Source: CAD feature listing. Evaluate the final solid. Frame: model axes, mm. A direction names the side the tool comes from. Round coordinates to 2 decimals unless told otherwise and drop trailing zeros. Write each loop counter-clockwise with the first axis right and the second up, starting at its lowest first coordinate (ties: lowest second). Pieces come first, ordered by that corner, then holes. Notation, with made-up numbers: M 46.25,65.5 L 97.25,65.5 A26 ccw 97.25,88.5 Z; hole C -32.5,70.5 d9. An arc over 180 degrees is marked long. Answer in a Markdown table with one row per item.
from build123d import *

# Parameters (mm, degrees)
SKETCH1_W               = 59.992800004
SKETCH1_H               = 59.7535
BOSS_EXTRUDE1_DEPTH     = 2.54
SKETCH2_R               = 2.286000002
BOSS_EXTRUDE2_DEPTH     = 4.7625
SKETCH3_R               = 1.270000002
CUT_EXTRUDE1_DEPTH      = 3.175
CUT_EXTRUDE2_REACH      = 44.962
SKETCH4_W               = 30.1625
SKETCH4_H               = 22.225
CUT_EXTRUDE3_REACH      = 44.962
SKETCH5_R               = 1.269999998
SKETCH6_W               = 38.1
SKETCH6_H               = 1.5875
BOSS_EXTRUDE3_DEPTH     = 3.175
CHAMFER1_SIZE           = 3.175
CUT_EXTRUDE4_DEPTH      = 43.603821541
CUT_EXTRUDE4_DEPTH_BACK = 43.603821541
CUT_EXTRUDE5_DEPTH      = 9.525
CUT_EXTRUDE5_DEPTH_BACK = 9.525
SKETCH8_R               = 1.5875
SKETCH9_W               = 5.588
SKETCH9_H               = 1.905
SKETCH9_W_2             = 5.08
CUT_EXTRUDE6_DEPTH      = 43.96196818
FILLET1_R               = 2.54


with BuildPart() as part:
    # Sketch1 → Boss-Extrude1 (new body)
    with BuildSketch(Plane.XY):
        Rectangle(SKETCH1_W, SKETCH1_H)
    extrude(amount=BOSS_EXTRUDE1_DEPTH)

    # Sketch2 → Boss-Extrude2 (add)
    with BuildSketch(Plane(origin=(0, 0, 0), x_dir=(-1, 0, 0), z_dir=(0, 0, -1))):
        with Locations(Location((-22.859000002, 22.60425, 0), (0, 0, 180))):
            Circle(SKETCH2_R)
        with Locations(Location((22.860999998, 21.93925, 0), (0, 0, 180))):
            Circle(SKETCH2_R)
        with Locations(Location((22.860999998, 4.15925, 0), (0, 0, 180))):
            Circle(SKETCH2_R)
        with Locations(Location((-22.859000002, 3.49425, 0), (0, 0, 180))):
            Circle(SKETCH2_R)
        with Locations(Location((-22.859000002, -4.12575, 0), (0, 0, 180))):
            Circle(SKETCH2_R)
        with Locations(Location((-2.539000002, -4.12575, 0), (0, 0, 180))):
            Circle(SKETCH2_R)
        with Locations(Location((-22.859000002, -21.90575, 0), (0, 0, 180))):
            Circle(SKETCH2_R)
        with Locations(Location((-2.539000002, -21.90575, 0), (0, 0, 180))):
            Circle(SKETCH2_R)
    extrude(amount=BOSS_EXTRUDE2_DEPTH)

    # Sketch3 → Cut-Extrude1 (cut)
    with BuildSketch(Plane(origin=(0, 0, -4.7625), x_dir=(-1, 0, 0), z_dir=(0, 0, -1))):
        with Locations((-22.859000002, 22.60425)):
            Circle(SKETCH3_R)
        with Locations((22.860999998, 21.93925)):
            Circle(SKETCH3_R)
        with Locations((22.860999998, 4.15925)):
            Circle(SKETCH3_R)
        with Locations((-2.539000002, -4.12575)):
            Circle(SKETCH3_R)
        with Locations((-22.859000002, 3.49425)):
            Circle(SKETCH3_R)
        with Locations((-22.859000002, -4.12575)):
            Circle(SKETCH3_R)
        with Locations((-22.859000002, -21.90575)):
            Circle(SKETCH3_R)
        with Locations((-2.539000002, -21.90575)):
            Circle(SKETCH3_R)
    extrude(amount=-CUT_EXTRUDE1_DEPTH, mode=Mode.SUBTRACT)

    # Sketch4 → Cut-Extrude2 (cut, up to next)
    with BuildSketch(Plane.XY.offset(2.54), mode=Mode.PRIVATE) as cut_extrude2_sk1:
        with Locations((-0.280399998, 13.21435)):
            Rectangle(SKETCH4_W, SKETCH4_H)
    cut_extrude2_tool1 = extrude(cut_extrude2_sk1.sketch, amount=-CUT_EXTRUDE2_REACH, mode=Mode.PRIVATE) & part.part
    add(cut_extrude2_tool1.solids().sort_by_distance((-0.2804, 13.21435, 2.54))[0], mode=Mode.SUBTRACT)

    # Sketch5 → Cut-Extrude3 (cut, up to next)
    with BuildSketch(Plane.XY.offset(2.54), mode=Mode.PRIVATE) as cut_extrude3_sk1:
        with Locations((-17.780999998, 20.03425)):
            Circle(SKETCH5_R)
    cut_extrude3_tool1 = extrude(cut_extrude3_sk1.sketch, amount=-CUT_EXTRUDE3_REACH, mode=Mode.PRIVATE) & part.part
    # Sketch5 → Cut-Extrude3 (cut, up to next)
    with BuildSketch(Plane.XY.offset(2.54), mode=Mode.PRIVATE) as cut_extrude3_sk2:
        with Locations((-17.780999998, 13.04925)):
            Circle(SKETCH5_R)
    cut_extrude3_tool2 = extrude(cut_extrude3_sk2.sketch, amount=-CUT_EXTRUDE3_REACH, mode=Mode.PRIVATE) & part.part
    # Sketch5 → Cut-Extrude3 (cut, up to next)
    with BuildSketch(Plane.XY.offset(2.54), mode=Mode.PRIVATE) as cut_extrude3_sk3:
        with Locations((-17.780999998, 6.06425)):
            Circle(SKETCH5_R)
    cut_extrude3_tool3 = extrude(cut_extrude3_sk3.sketch, amount=-CUT_EXTRUDE3_REACH, mode=Mode.PRIVATE) & part.part
    # Sketch5 → Cut-Extrude3 (cut, up to next)
    with BuildSketch(Plane.XY.offset(2.54), mode=Mode.PRIVATE) as cut_extrude3_sk4:
        with Locations((19.049000002, 13.04925)):
            Circle(SKETCH5_R)
    cut_extrude3_tool4 = extrude(cut_extrude3_sk4.sketch, amount=-CUT_EXTRUDE3_REACH, mode=Mode.PRIVATE) & part.part
    add(cut_extrude3_tool1.solids().sort_by_distance((-17.781, 20.03425, 2.54))[0], mode=Mode.SUBTRACT)
    add(cut_extrude3_tool2.solids().sort_by_distance((-17.781, 13.04925, 2.54))[0], mode=Mode.SUBTRACT)
    add(cut_extrude3_tool3.solids().sort_by_distance((-17.781, 6.06425, 2.54))[0], mode=Mode.SUBTRACT)
    add(cut_extrude3_tool4.solids().sort_by_distance((19.049, 13.04925, 2.54))[0], mode=Mode.SUBTRACT)

    # Sketch6 → Boss-Extrude3 (add)
    with BuildSketch(Plane(origin=(0, 0, 0), x_dir=(-1, 0, 0), z_dir=(0, 0, -1))):
        with Locations((0, 25.81275)):
            Rectangle(SKETCH6_W, SKETCH6_H)
        with Locations((0, -25.81275)):
            Rectangle(SKETCH6_W, SKETCH6_H)
    extrude(amount=BOSS_EXTRUDE3_DEPTH)

    # Chamfer1
    chamfer1_edges = [part.edges().sort_by_distance(p)[0] for p in [
        (29.996400002, -29.87675, 1.27),
        (-29.996400002, -29.87675, 1.27),
        (-29.996400002, 29.87675, 1.27),
        (29.996400002, 29.87675, 1.27),
    ]]
    chamfer(chamfer1_edges, length=CHAMFER1_SIZE)

    # Sketch7 → Cut-Extrude4 (cut, two sides: drawn at the far end of the back side and taken through both)
    with BuildSketch(Plane(origin=(0, 0, 0), x_dir=(0, 0, -1), z_dir=(1, 0, 0)).offset(-CUT_EXTRUDE4_DEPTH_BACK)):
        with BuildLine():
            Line((0, 26.6065), (0.5, 26.6065))
            ThreePointArc((0.5, 26.6065), (0.25, 26.3565), (0, 26.6065))
        make_face()
        with BuildLine():
            Line((0, -26.6065), (0.5, -26.6065))
            ThreePointArc((0.5, -26.6065), (0.25, -26.3565), (0, -26.6065))
        make_face()
    extrude(amount=CUT_EXTRUDE4_DEPTH + CUT_EXTRUDE4_DEPTH_BACK, mode=Mode.SUBTRACT)

    # Sketch8 → Cut-Extrude5 (cut, two sides: drawn at the far end of the back side and taken through both)
    with BuildSketch(Plane(origin=(0, 0, 0), x_dir=(0, 0, -1), z_dir=(1, 0, 0)).offset(-CUT_EXTRUDE5_DEPTH_BACK)):
        with Locations((0, 29.87675)):
            Circle(SKETCH8_R)
        with Locations((0, -29.87675)):
            Circle(SKETCH8_R)
    extrude(amount=CUT_EXTRUDE5_DEPTH + CUT_EXTRUDE5_DEPTH_BACK, mode=Mode.SUBTRACT)

    # Sketch9 → Cut-Extrude6 (cut, through all)
    with BuildSketch(Plane.XY.offset(2.54)):
        with Locations((17.594850002, 3.05435)):
            Rectangle(SKETCH9_W, SKETCH9_H)
        with Locations((-17.901649998, 23.37435)):
            Rectangle(SKETCH9_W_2, SKETCH9_H)
        with Locations((17.594850002, 23.37435)):
            Rectangle(SKETCH9_W, SKETCH9_H)
    extrude(amount=-CUT_EXTRUDE6_DEPTH, mode=Mode.SUBTRACT)

    # Fillet1
    fillet1_edges = [part.edges().sort_by_distance(p)[0] for p in [
        (14.800850002, 4.00685, 1.27),
        (-15.361649998, 22.42185, 1.27),
        (14.800850002, 22.42185, 1.27),
        (-15.361649998, 2.10185, 1.27),
    ]]
    fillet(fillet1_edges, radius=FILLET1_R)


solid = part.part
Q1. Pull-direction query (Y, two-part tool) for faces 1 (the flat face through (0, -26.606, -2)), 2 (the flat face through (-9.525, -29, 1)), 3 (the flat face through (0, 24.327, 1)); classes: pulls with the +Y half, pulls with the -Y half, needs draft (parallel to the pull), parting line crosses it, or undercut.
Solutions:
| item | result |
|---|---|
| face 1 | pulls with the -Y half |
| face 2 | needs draft |
| face 3 | undercut |
Q2. Section B-B (y = 9). Return loops of the section in (x, z).
Solutions:
| item | result |
|---|---|
| outline | M -30,0 L -15.36,0 L -15.36,2.54 L -30,2.54 Z; M 14.8,0 L 30,0 L 30,2.54 L 14.8,2.54 Z |
Q3. Access query for faces 4 (the flat face through (20.389, 23, 1)), 5 (the flat face through (0, -25.019, -2)), 6 (the cylindrical face through (22.363, 24.836, -2.348)), 7 (the cylindrical face through (-0.13, -28.74, 1.11)). Directions: +Z, -Z, +X, -X, +Y, -Y. A direction counts if a zero-diameter tool reaches every point of the face in a straight line with its end or side. Return the directions, or none.
Solutions:
| item | result |
|---|---|
| face 4 | +Z, -Z |
| face 5 | -Z, +X, -X |
| face 6 | -Z |
| face 7 | -Z, -Y |
Q4. Material intervals for probe 1 along Y at (x, z) = (21.5, -3.5); probe 2 along Y at (x, z) = (-19, -2.25); probe 3 along Y at (x, z) = (12.5, -0.25), sorted ascending.
Solutions:
| item | result |
|---|---|
| probe 1 | y = -23.74 to -20.07, -5.96 to -2.29, 1.66 to 5.33, 20.77 to 24.44 |
| probe 2 | y = -26.61 to -25.02, 25.02 to 26.61 |
| probe 3 | y = -26.36 to -25.02, 25.02 to 26.36 |
Q5. Contact query for flat-ended pins moving along their axis: pin 1 Ø1 at (x, z) = (17, -4) entering from +Y; pin 2 Ø0.8 at (x, y) = (23, -22) entering from -Z; pin 3 Ø1.6 at (x, z) = (5, -1) entering from -Y; pin 4 Ø1.5 at (x, z) = (-21, -2) entering from +Y. Output: stop coordinate, or through.
Solutions:
| item | result |
|---|---|
| pin 1 | passes through |
| pin 2 | stops at z = -1.59 |
| pin 3 | stops at y = -26.61 |
| pin 4 | stops at y = 23.94 |
